Check sheet for the drawn part. Datum: minimum x, y, z corner. Units: mm. Coordinates: 2 decimals unless noted, no trailing zeros. Loops run counter-clockwise (first coordinate to the right, second up) from the corner with the lowest first, then second, coordinate; pieces in that order, holes last. Notation, with made-up numbers: (49.5, -31.5) -> (104.5, -31.5) arc R34 cw to (104.5, 1.5) -> close; hole circle Ø4 at (-32, -38). An arc over 180 degrees is marked (long way). Use CSV: the item, a comma, the result in double quotes. Start each with the question number.
1. Sectioned sample at D-D, the plane y = 7.25. Record the cut outline in (x, z).
2. Sectioned sample at C-C, the plane x = 66.5. Record the cut outline in (y, z).
3. Sectioned sample at B-B, the plane z = 7.75. Record the cut outline in (x, y).
4. Release check for a two-part mould opening along Y. For the marked faces 1, 2, 3 and 4 record: pulls with the +Y half, pulls with the -Y half, needs draft (parallel to the pull), parting line crosses it, or undercut.
5. Thickness scan on L1, parallel to X at y = 14.2, z = 5; L2, parallel to Y at x = 50, z = 4.25; L3, parallel to Z at x = 5, y = 14.45. Record the ranges inside material, lowest first.
6. Sectioned sample at A-A, the plane x = 101. Record the cut outline in (y, z).
7. Gauge pin test, flat ends, axial feed: pin 1 (3 mm diameter, centred on x = 101, z = 5, fed in from -Y); pin 2 (3.5 mm diameter, centred on x = 5, z = 5, fed in from -Y). Record the tip position at first contact, or that the pin passes through.
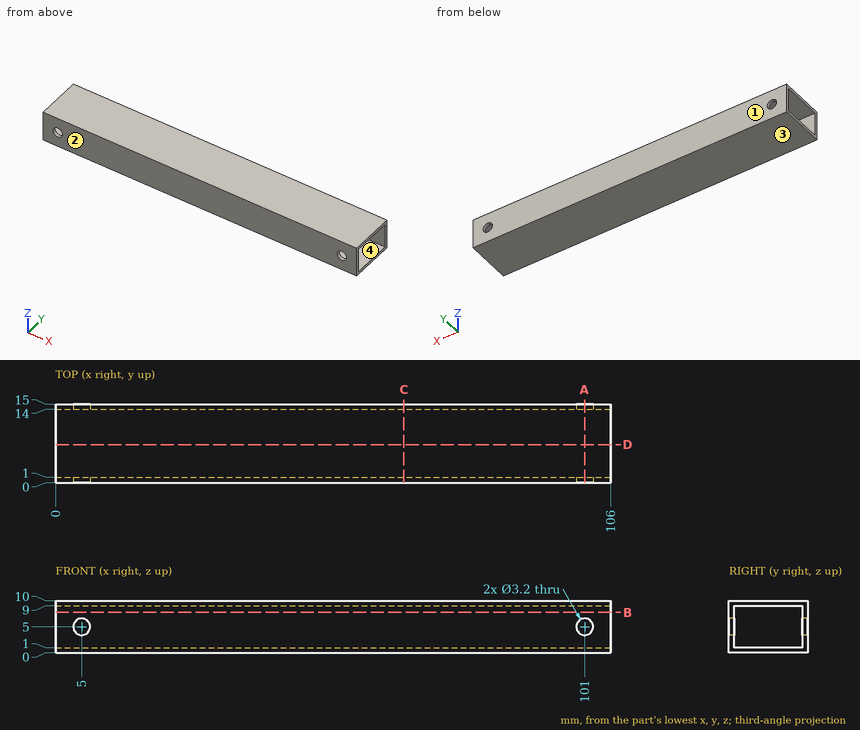
Completed:
1,outline,"(0, 0) -> (106, 0) -> (106, 1) -> (0, 1) -> close; (0, 9) -> (106, 9) -> (106, 10) -> (0, 10) -> close"
2,outline,"(0, 0) -> (15, 0) -> (15, 10) -> (0, 10) -> close; hole (1, 1) -> (14, 1) -> (14, 9) -> (1, 9) -> close"
3,outline,"(0, 0) -> (106, 0) -> (106, 1) -> (0, 1) -> close; (0, 14) -> (106, 14) -> (106, 15) -> (0, 15) -> close"
4,face 1,"pulls with the +Y half"
4,face 2,"pulls with the -Y half"
4,face 3,"needs draft"
4,face 4,"undercut"
5,L1,"0 to 3.4, 6.6 to 99.4, 102.6 to 106"
5,L2,"0 to 1, 14 to 15"
5,L3,"0 to 3.4, 6.6 to 10"
6,outline,"(0, 0) -> (15, 0) -> (15, 3.4) -> (14, 3.4) -> (14, 1) -> (1, 1) -> (1, 3.4) -> (0, 3.4) -> close; (0, 6.6) -> (1, 6.6) -> (1, 9) -> (14, 9) -> (14, 6.6) -> (15, 6.6) -> (15, 10) -> (0, 10) -> close"
7,pin 1,"through"
7,pin 2,"y = 0"
